Work out the finished part from the listing and answer in its coordinate system (mm). Face numbers are marked on the shaded views. A direction names the side the tool comes from. Give positions to 0.01 mm unless a question says otherwise; leave off trailing zeros. Loops run counter-clockwise (first coordinate to the right, second up) from the corner with the lowest first, then second, coordinate; pieces in that order, holes last. Notation, with made-up numbers: (83.25, -33.75) - (98.25, -33.75) arc R25 ccw to (98.25, -13.75) - close; hole circle Ø3 at (72.25, 32). An arc over 180 degrees is marked (long way). One line per item, written item: value.
from build123d import *

# Parameters (mm, degrees)
CYLINDER001_R     = 2.1
CYLINDER001_DEPTH = 10
BOX004_W          = 16
BOX004_H          = 6
BOX004_DEPTH      = 11
BOX003_W          = 9
BOX003_H          = 11
BOX003_DEPTH      = 11
BOX002_W          = 22
BOX002_H          = 3
BOX002_DEPTH      = 11
BOX001_W          = 3
BOX001_H          = 25
BOX001_DEPTH      = 11
CYLINDER_R        = 2
CYLINDER_DEPTH    = 10
BOX_W             = 26
BOX_H             = 13
BOX_DEPTH         = 23
BOX_ROLL_ANGLE    = 90
CHAMFER_SIZE      = 1
CHAMFER001_SIZE   = 1
CHAMFER002_SIZE   = 1


with BuildPart() as cylinder001:
    # Cylinder001 → Cylinder001 (new body)
    with BuildSketch(Plane(origin=(5, -5, -5), x_dir=(1, 0, 0), z_dir=(0, 0, 1))):
        Circle(CYLINDER001_R)
    extrude(amount=CYLINDER001_DEPTH)


with BuildPart() as cube004:
    # Box004 → Box004 (new body)
    with BuildSketch(Plane(origin=(2, -15, -1), x_dir=(1, 0, 0), z_dir=(0, 0, 1))):
        with Locations((8, 3)):
            Rectangle(BOX004_W, BOX004_H)
    extrude(amount=BOX004_DEPTH)


with BuildPart() as cube003:
    # Box003 → Box003 (new body)
    with BuildSketch(Plane(origin=(9, -13, -1), x_dir=(1, 0, 0), z_dir=(0, 0, 1))):
        with Locations((4.5, 5.5)):
            Rectangle(BOX003_W, BOX003_H)
    extrude(amount=BOX003_DEPTH)


with BuildPart() as cube002:
    # Box002 → Box002 (new body)
    with BuildSketch(Plane(origin=(-1, -20, -1), x_dir=(1, 0, 0), z_dir=(0, 0, 1))):
        with Locations((11, 1.5)):
            Rectangle(BOX002_W, BOX002_H)
    extrude(amount=BOX002_DEPTH)


with BuildPart() as cube001:
    # Box001 → Box001 (new body)
    with BuildSketch(Plane(origin=(20, -24, -1), x_dir=(1, 0, 0), z_dir=(0, 0, 1))):
        with Locations((1.5, 12.5)):
            Rectangle(BOX001_W, BOX001_H)
    extrude(amount=BOX001_DEPTH)


with BuildPart() as cylinder:
    # Cylinder → Cylinder (new body)
    with BuildSketch(Plane(origin=(5, -5, -5), x_dir=(1, 0, 0), z_dir=(0, 0, 1))):
        Circle(CYLINDER_R)
    extrude(amount=CYLINDER_DEPTH)


with BuildPart() as cut005:
    # Box → Box (new body)
    with BuildSketch(Plane.XY):
        with Locations((13, 6.5)):
            Rectangle(BOX_W, BOX_H)
    extrude(amount=BOX_DEPTH)


with BuildPart() as cut005_1:
    # Box roll: moved
    add(cut005.part.rotate(Axis((0, 0, 0), (1, 0, 0)), BOX_ROLL_ANGLE))


with BuildPart() as cut005_2:
    # Box placement: moved
    add(cut005_1.part)

    # Cut: cut Cylinder
    add(cylinder.part, mode=Mode.SUBTRACT)

    # Cut001: cut Cube001
    add(cube001.part, mode=Mode.SUBTRACT)

    # Cut002: cut Cube002
    add(cube002.part, mode=Mode.SUBTRACT)

    # Cut003: cut Cube003
    add(cube003.part, mode=Mode.SUBTRACT)

    # Cut004: cut Cube004
    add(cube004.part, mode=Mode.SUBTRACT)

    # Chamfer
    chamfer_edges = [cut005_2.edges().sort_by_distance(p)[0] for p in [
        (20, -8.5, 0),
        (10, -17, 0),
        (10, -20, 0),
        (20, -21.5, 0),
        (23, -11.5, 0),
    ]]
    chamfer(chamfer_edges, length=CHAMFER_SIZE)

    # Chamfer001
    chamfer001_edges = [cut005_2.edges().sort_by_distance(p)[0] for p in [
        (0, -8, 0),
        (0, -22, 0),
        (9.5, 0, 0),
        (25, 0, 0),
        (25, -23, 0),
        (9.5, -23, 0),
        (26, -11.5, 0),
    ]]
    chamfer(chamfer001_edges, length=CHAMFER001_SIZE)

    # Chamfer002
    chamfer002_edges = [cut005_2.edges().sort_by_distance(p)[0] for p in [
        (0, -11.5, 13),
        (13, 0, 13),
        (26, -11.5, 13),
        (13, -23, 13),
    ]]
    chamfer(chamfer002_edges, length=CHAMFER002_SIZE)

    # Cut005: cut Cylinder001
    add(cylinder001.part, mode=Mode.SUBTRACT)


solid = cut005_2.part
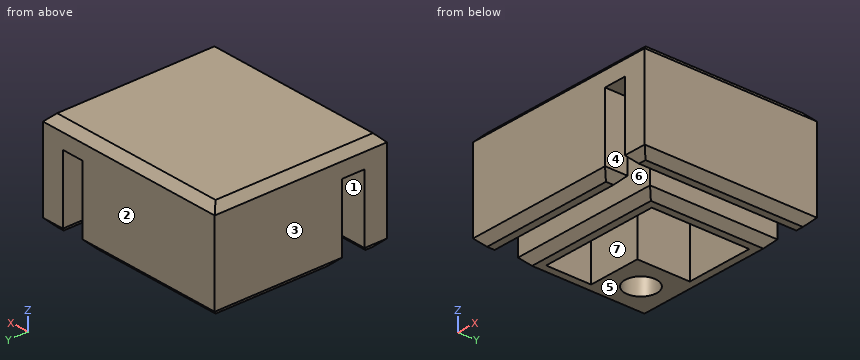
1. Section D-D (x = 21) is taken. Write down the section's boundary in (y, z).
Output:
outline: (-23, 10) - (0, 10) - (0, 12) - (-1, 13) - (-22, 13) - (-23, 12) - close
2. Find the intervals of material crossed by line 1 along X through (y, z) = (-8.5, 4.5); line 2 along Y through (x, z) = (10.5, 6); line 3 along Y through (x, z) = (5, 1.55), in increasing order.
Output:
line 1: x = 0 to 9, 18 to 20, 23 to 26
line 2: y = -23 to -20, -17 to -15, -2 to 0
line 3: y = -23 to -20, -17 to -15, -9 to -7.1, -2.9 to 0
3. Flat-ended cylindrical pins translate along their axes: pin 1 Ø4 at (x, y) = (11.5, -10.5) entering from -Z; pin 2 Ø1.3 at (x, y) = (6, -4.5) entering from -Z. Find the tip coordinate at first contact, or state that the pin passes through.
Output:
pin 1: stops at z = 10
pin 2: stops at z = 5
4. For the marked faces 4, 5, 6 and 7, determine the directions among +Z, -Z, +X, -X, +Y, -Y from which every point of the face is accessible in a straight line to the end or side of a thin tool.
Output:
face 4: -Z, +Y, -Y
face 5: -Z, +X, -X, +Y, -Y
face 6: -Z, -X
face 7: -Z
5. Section C-C (y = -5) is taken. Write down the section's boundary in (x, z).
Output:
outline: (0, 1) - (1, 0) - (2.9, 0) - (2.9, 5) - (7.1, 5) - (7.1, 0) - (9, 0) - (9, 10) - (18, 10) - (18, 0) - (19, 0) - (20, 1) - (20, 10) - (23, 10) - (23, 1) - (24, 0) - (25, 0) - (26, 1) - (26, 12) - (25, 13) - (1, 13) - (0, 12) - close
6. Section B-B (x = 5) is taken. Write down the section's boundary in (y, z), and give its area (3 significant figures).
Output:
outline: (-23, 1) - (-22, 0) - (-21, 0) - (-20, 1) - (-20, 10) - (-17, 10) - (-17, 1) - (-16, 0) - (-15, 0) - (-15, 10) - (-9, 10) - (-9, 0) - (-7.1, 0) - (-7.1, 5) - (-2.9, 5) - (-2.9, 0) - (-1, 0) - (0, 1) - (0, 12) - (-1, 13) - (-22, 13) - (-23, 12) - close
area: 185 mm²
7. Section A-A (z = 3) is taken. Write down the section's boundary in (x, y), and give its area (3 significant figures).
Output:
outline: (0, -23) - (20, -23) - (20, -20) - (0, -20) - close; (0, -17) - (20, -17) - (20, 0) - (0, 0) - close; (23, -23) - (26, -23) - (26, 0) - (23, 0) - close; hole (2, -15) - (18, -15) - (18, -2) - (9, -2) - (9, -9) - (2, -9) - close; hole circle Ø4.2 at (5, -5)
area: 296 mm²
8. The mould has two halves that part along Y. Classify the marked faces 1, 2 and 3: released by +Y, released by -Y, zero draft, split by the parting line, or undercut.
Output:
face 1: undercut
face 2: released by +Y
face 3: zero draft
